Check sheet for the modelled part. Datum: model origin and axes. Units: mm. Round coordinates to 2 decimals unless told otherwise and drop trailing zeros. Order: outer loops, then holes, each group sorted by start corner. A loop starts at its lowest first (then second) coordinate and runs counter-clockwise, first axis right, second up.
```python
from build123d import *

# Parameters (mm, degrees)
BOSS_EXTRUDE1_DEPTH = 3.175


with BuildPart() as part:
    # Sketch1 → Boss-Extrude1 (new body)
    with BuildSketch(Plane(origin=(0, 0, 0), x_dir=(1, 0, 0), z_dir=(0, 1, 0))):
        with BuildLine():
            Line((3.175, 0), (13, 0))
            Line((13, 0), (13.75, -13))
            Line((13.75, -13), (14.5, 0))
            Line((14.5, 0), (16, 0))
            Line((16, 0), (16.75, -13))
            Line((16.75, -13), (17.5, 0))
            Line((17.5, 0), (19, 0))
            Line((19, 0), (19.75, -13))
            Line((19.75, -13), (20.5, 0))
            Line((20.5, 0), (22, 0))
            Line((22, 0), (22.75, -13))
            Line((22.75, -13), (23.5, 0))
            Line((23.5, 0), (25, 0))
            Line((25, 0), (25.75, -13))
            Line((25.75, -13), (26.5, 0))
            Line((26.5, 0), (28, 0))
            Line((28, 0), (28.75, -13))
            Line((28.75, -13), (29.5, 0))
            Line((29.5, 0), (31, 0))
            Line((31, 0), (31.75, -13))
            Line((31.75, -13), (32.5, 0))
            Line((32.5, 0), (34, 0))
            Line((34, 0), (34.75, -13))
            Line((34.75, -13), (35.5, 0))
            Line((35.5, 0), (37, 0))
            Line((37, 0), (37.75, -13))
            Line((37.75, -13), (38.5, 0))
            Line((38.5, 0), (40, 0))
            Line((40, 0), (41, 0))
            Line((41, 0), (41, -30))
            Line((41, -30), (40, -30))
            Line((40, -30), (38.5, -30))
            Line((38.5, -30), (37.75, -17))
            Line((37.75, -17), (37, -30))
            Line((37, -30), (35.5, -30))
            Line((35.5, -30), (34.75, -17))
            Line((34.75, -17), (34, -30))
            Line((34, -30), (32.5, -30))
            Line((32.5, -30), (31.75, -17))
            Line((31.75, -17), (31, -30))
            Line((31, -30), (29.5, -30))
            Line((29.5, -30), (28.75, -17))
            Line((28.75, -17), (28, -30))
            Line((28, -30), (26.5, -30))
            Line((26.5, -30), (25.75, -17))
            Line((25.75, -17), (25, -30))
            Line((25, -30), (23.5, -30))
            Line((23.5, -30), (22.75, -17))
            Line((22.75, -17), (22, -30))
            Line((22, -30), (20.5, -30))
            Line((20.5, -30), (19.75, -17))
            Line((19.75, -17), (19, -30))
            Line((19, -30), (17.5, -30))
            Line((17.5, -30), (16.75, -17))
            Line((16.75, -17), (16, -30))
            Line((16, -30), (14.5, -30))
            Line((14.5, -30), (13.75, -17))
            Line((13.75, -17), (13, -30))
            Line((13, -30), (3.175, -30))
            Line((3.175, -30), (3.175, -20))
            Line((3.175, -20), (0, -20))
            Line((0, -20), (0, -15.871779789))
            ThreePointArc((0, -15.871779789), (3.8, -15), (0, -14.128220211))
            Line((0, -14.128220211), (0, -10))
            Line((0, -10), (3.175, -10))
            Line((3.175, -10), (3.175, 0))
        make_face()
        Polygon((15.25, -2), (16, -15), (15.25, -28), (14.5, -15), align=None, mode=Mode.SUBTRACT)
        Polygon((18.25, -2), (17.5, -15), (18.25, -28), (19, -15), align=None, mode=Mode.SUBTRACT)
        Polygon((21.25, -2), (20.5, -15), (21.25, -28), (22, -15), align=None, mode=Mode.SUBTRACT)
        Polygon((24.25, -2), (23.5, -15), (24.25, -28), (25, -15), align=None, mode=Mode.SUBTRACT)
        Polygon((27.25, -2), (26.5, -15), (27.25, -28), (28, -15), align=None, mode=Mode.SUBTRACT)
        Polygon((30.25, -2), (29.5, -15), (30.25, -28), (31, -15), align=None, mode=Mode.SUBTRACT)
        Polygon((33.25, -2), (32.5, -15), (33.25, -28), (34, -15), align=None, mode=Mode.SUBTRACT)
        Polygon((36.25, -2), (35.5, -15), (36.25, -28), (37, -15), align=None, mode=Mode.SUBTRACT)
        Polygon((39.25, -2), (38.5, -15), (39.25, -28), (40, -15), align=None, mode=Mode.SUBTRACT)
    extrude(amount=BOSS_EXTRUDE1_DEPTH)


solid = part.part
```
Item 1: Sectioned sample at A-A (x = 1.8). Record the cut outline in (y, z) (3 decimals).
Answer:
outline: (0, 10) - (3.175, 10) - (3.175, 13) - (0, 13) - close; (0, 17) - (3.175, 17) - (3.175, 20) - (0, 20) - close
Item 2: Sectioned sample at B-B (y = 0.6). State how many separate pieces and enclosed holes the cut face has, and give its area (3 significant figures).
Answer:
separate pieces: 1
enclosed holes: 9
area: 803 mm2
Item 3: Go/stop test with flat-tipped pins: P1, Ø1.6, axis at x = 2, y = 2, coming from the +Z side; P2, Ø1.6, axis at y = 1, z = 4.5, coming from the -X side (3 decimals); P3, Ø3.5, axis at x = 1.8, z = 15, coming from the -Y side (3 decimals). Record where each tip stops, or that it passes through.
Answer:
P1: stops at z = 20
P2: stops at x = 3.175
P3: passes through
Item 4: Scan line: line 1 along Z through (x, y) = (1.8, 0.7). Record every from-to range of solid material in increasing order.
Answer:
line 1: z = 10 to 13, 17 to 20
Item 5: Release check for a two-part mould opening along Z. For faces 1 (the flat face through (36, 2, 0)), 2 (the flat face through (32.87, 1.57, 21.41)), 3 (the flat face through (0, 2, 12)) record: released by +Z, released by -Z, zero draft, split by the parting line, or undercut.
Answer:
face 1: released by -Z
face 2: undercut
face 3: zero draft
